Geometry: final body of the model. Coordinates: model frame, mm. A direction names the side the tool comes from. Give positions to 0.01 mm unless a question says otherwise; leave off trailing zeros. Loops run counter-clockwise (first coordinate to the right, second up) from the corner with the lowest first, then second, coordinate; pieces in that order, holes last. Notation, with made-up numbers: (-14.5, -36.5) - (-0.5, -36.5) arc R8 ccw to (-0.5, -26.5) - close; hole circle Ø9 at (8.5, 6). An arc over 180 degrees is marked (long way). Use one line per item in the form item = value.
```python
from build123d import *

# Parameters (mm, degrees)
BOSS_EXTRUDE1_DEPTH = 31.75
SKETCH2_R           = 3.175
CUT_EXTRUDE1_DEPTH  = 195.587542385


with BuildPart() as part:
    # Sketch1 → Boss-Extrude1 (new, symmetric)
    with BuildSketch(Plane(origin=(0, 0, 0), x_dir=(1, 0, 0), z_dir=(0, 1, 0))):
        with BuildLine():
            ThreePointArc((119.54162455, 19.05), (0, 121.05), (-119.54162455, 19.05))
            Line((-119.54162455, 19.05), (-158.481944244, 19.05))
            Line((-158.481944244, 19.05), (-158.481944244, 12.7))
            Line((-158.481944244, 12.7), (-120.381944244, 12.7))
            Line((-120.381944244, 12.7), (-113.994736721, 12.7))
            ThreePointArc((-113.994736721, 12.7), (0, 114.7), (113.994736721, 12.7))
            Line((113.994736721, 12.7), (120.381944244, 12.7))
            Line((120.381944244, 12.7), (158.481944244, 12.7))
            Line((158.481944244, 12.7), (158.481944244, 19.05))
            Line((158.481944244, 19.05), (119.54162455, 19.05))
        make_face()
    extrude(amount=BOSS_EXTRUDE1_DEPTH, both=True)

    # Sketch2 → Cut-Extrude1 (cut, through all)
    with BuildSketch(Plane.XY.offset(-12.7)):
        with Locations((-129.276704473, 15.875)):
            Circle(SKETCH2_R)
        with Locations((-148.746864321, 15.875)):
            Circle(SKETCH2_R)
        with Locations((-148.746864321, -15.875)):
            Circle(SKETCH2_R)
        with Locations((-129.276704473, -15.875)):
            Circle(SKETCH2_R)
        with Locations((129.276704473, 15.875)):
            Circle(SKETCH2_R)
        with Locations((148.746864321, 15.875)):
            Circle(SKETCH2_R)
        with Locations((129.276704473, -15.875)):
            Circle(SKETCH2_R)
        with Locations((148.746864321, -15.875)):
            Circle(SKETCH2_R)
    extrude(amount=-CUT_EXTRUDE1_DEPTH, mode=Mode.SUBTRACT)


solid = part.part
```
(1) Pin query (flat end, axial travel): P1, Ø5, axis at y = 13.5, z = -49, coming from the +X side; P2, Ø10, axis at x = 148.75, y = -15.88, coming from the -Z side; P3, Ø4, axis at x = -148.75, y = -15.88, coming from the -Z side; P4, Ø5, axis at y = 7, z = -96.5, coming from the +X side. Return the tip coordinate at first contact, or that it passes through.
Solution:
P1 = 111.76
P2 = -19.05
P3 = through
P4 = 76.27
(2) Cut plane B-B (z = -52). Return the cut outline in (x, y), plus the area to 3 significant figures.
Solution:
outline = (-109.31, -31.75) - (-102.24, -31.75) - (-102.24, 31.75) - (-109.31, 31.75) - close; (102.24, -31.75) - (109.31, -31.75) - (109.31, 31.75) - (102.24, 31.75) - close
area = 899 mm2
(3) Material intervals for L1, parallel to X at y = 2.5, z = -91.5; L2, parallel to X at y = 12, z = -40; L3, parallel to Z at x = -134, y = 29, sorted ascending. Write a range as from..to.
Solution:
L1 = -79.25..-69.17, 69.17..79.25
L2 = -114.25..-107.5, 107.5..114.25
L3 = -19.05..-12.7
(4) Cut plane D-D (x = 90.5). Return the cut outline in (y, z).
Solution:
outline = (-31.75, -80.39) - (31.75, -80.39) - (31.75, -70.47) - (-31.75, -70.47) - close
(5) Cut plane C-C (z = -22). Return the cut outline in (x, y), plus the area to 3 significant figures.
Solution:
outline = (-119.03, -31.75) - (-112.57, -31.75) - (-112.57, 31.75) - (-119.03, 31.75) - close; (112.57, -31.75) - (119.03, -31.75) - (119.03, 31.75) - (112.57, 31.75) - close
area = 821 mm2
(6) Cut plane A-A (y = -24.5). Return the cut outline in (x, z), plus the area to 3 significant figures.
Solution:
outline = (-158.48, -19.05) - (-119.54, -19.05) arc R121.05 ccw to (119.54, -19.05) - (158.48, -19.05) - (158.48, -12.7) - (113.99, -12.7) arc R114.7 cw to (-113.99, -12.7) - (-158.48, -12.7) - close
area = 2,680 mm2
(7) Access query for faces 1 (the face through (-139, 0, -19.05)), 2 (the face through (-151.92, 16.01, -15.83)), 3 (the face through (139, 0, -19.05)). Directions: +Z, -Z, +X, -X, +Y, -Y. A direction counts if a zero-diameter tool reaches every point of the face in a straight line with its end or side. Return the directions, or none.
Solution:
face_1 = -Z, -X, +Y, -Y
face_2 = +Z, -Z
face_3 = -Z, +X, +Y, -Y
(8) Pull-direction query (X, two-part tool) for faces 4 (the face through (-1, 31.75, -115)), 5 (the face through (2.394, 0.444, -121.026)), 6 (the face through (-151.92, -15.74, -15.83)); classes: released by +X, released by -X, zero draft, split by the parting line, or undercut.
Solution:
face_4 = zero draft
face_5 = split by the parting line
face_6 = undercut
